Can you work these out from the model? Positions are in its coordinate system, mm. A direction names the side the tool comes from. Give positions to 0.01 mm unless a question says otherwise; leave off trailing zeros. Loops run counter-clockwise (first coordinate to the right, second up) from the corner with the lowest first, then second, coordinate; pieces in that order, holes last. Notation, with made-up numbers: (62.25, 26) -> (84.25, 26) arc R15 ccw to (84.25, 43) -> close; hole circle Ø2 at (11.25, 39). An arc over 180 degrees is marked (long way). One line per question, with ' | ' between items.
from build123d import *

# Parameters (mm, degrees)
SKETCH1_W             = 30
SKETCH1_H             = 30
SKETCH1_W_2           = 20
SKETCH1_H_2           = 20
BOSS_EXTRUDE1_DEPTH   = 20
BOSS_EXTRUDE2_START   = 20
SKETCH1_2_W           = 30
SKETCH1_2_H           = 30
SKETCH1_2_W_2         = 20
SKETCH1_2_H_2         = 20
BOSS_EXTRUDE2_DEPTH   = 10
SKETCH3_R             = 2.5
CUT_EXTRUDE1_DEPTH    = 46
SKETCH3_3_R           = 4
SKETCH3_3_R_2         = 2.5
CUT_EXTRUDE2_DEPTH    = 3
CUT_EXTRUDE3_START    = -27
SKETCH3_4_R           = 4
SKETCH3_4_R_2         = 2.5
CUT_EXTRUDE3_DEPTH    = 3
BOSS_EXTRUDE4_DEPTH   = 5
FILLET2_R             = 15
SKETCH7_R             = 2.5
CUT_EXTRUDE5_DEPTH    = 105.74180253
CRVPATTERN1_START     = -5
CRVPATTERN1_OUTLINE_R = 2.5
CRVPATTERN1_DEPTH     = 10


# Read off the part's stored shape, not the designer's step: CrvPattern1
with BuildPart() as part:
    # Sketch1 → Boss-Extrude1 (new body)
    with BuildSketch(Plane(origin=(0, 0, 0), x_dir=(1, 0, 0), z_dir=(0, 1, 0))):
        Rectangle(SKETCH1_W, SKETCH1_H)
        Rectangle(SKETCH1_W_2, SKETCH1_H_2, mode=Mode.SUBTRACT)
    extrude(amount=BOSS_EXTRUDE1_DEPTH)

    # Sketch1<2> → Boss-Extrude2 (add)
    # profile 1 of 2: a face of its own
    with BuildSketch(Plane(origin=(0, 0, 0), x_dir=(1, 0, 0), z_dir=(0, 1, 0)).offset(BOSS_EXTRUDE2_START)):
        Rectangle(SKETCH1_2_W, SKETCH1_2_H)
        Rectangle(SKETCH1_2_W_2, SKETCH1_2_H_2, mode=Mode.SUBTRACT)
    # profile 2 of 2: a face of its own
    with BuildSketch(Plane(origin=(0, 0, 0), x_dir=(1, 0, 0), z_dir=(0, 1, 0)).offset(BOSS_EXTRUDE2_START)):
        Rectangle(SKETCH1_2_W_2, SKETCH1_2_H_2)
    extrude(amount=BOSS_EXTRUDE2_DEPTH)

    # Sketch3 → Cut-Extrude1 (cut, through all)
    with BuildSketch(Plane(origin=(15, 0, 0), x_dir=(0, 0, -1), z_dir=(1, 0, 0))):
        with Locations((0, 15)):
            Circle(SKETCH3_R)
    extrude(amount=-CUT_EXTRUDE1_DEPTH, mode=Mode.SUBTRACT)

    # Sketch3<3> → Cut-Extrude2 (cut)
    # profile 1 of 2: a face of its own
    with BuildSketch(Plane(origin=(15, 0, 0), x_dir=(0, 0, -1), z_dir=(1, 0, 0))):
        Polygon((-5, 17.886751346), (-5, 12.113248654), (0, 9.226497308), (5, 12.113248654), (5, 17.886751346), (0, 20.773502692), align=None)
        with Locations((0, 15)):
            Circle(SKETCH3_3_R, mode=Mode.SUBTRACT)
    # profile 2 of 2: a face of its own
    with BuildSketch(Plane(origin=(15, 0, 0), x_dir=(0, 0, -1), z_dir=(1, 0, 0))):
        with Locations((0, 15)):
            Circle(SKETCH3_3_R)
        with Locations((0, 15)):
            Circle(SKETCH3_3_R_2, mode=Mode.SUBTRACT)
    extrude(amount=-CUT_EXTRUDE2_DEPTH, mode=Mode.SUBTRACT)

    # Sketch3<4> → Cut-Extrude3 (cut)
    with BuildSketch(Plane(origin=(15, 0, 0), x_dir=(0, 0, -1), z_dir=(1, 0, 0)).offset(CUT_EXTRUDE3_START)):
        with Locations((0, 15)):
            Circle(SKETCH3_4_R)
        with Locations((0, 15)):
            Circle(SKETCH3_4_R_2, mode=Mode.SUBTRACT)
    extrude(amount=-CUT_EXTRUDE3_DEPTH, mode=Mode.SUBTRACT)

    # Sketch6 → Boss-Extrude4 (add, symmetric)
    with BuildSketch(Plane(origin=(0, 0, 0), x_dir=(0, 0, -1), z_dir=(1, 0, 0))):
        Polygon((-15, 30), (-15, 100), (25.559724605, 100), (15, 0), (15, 30), align=None)
    extrude(amount=BOSS_EXTRUDE4_DEPTH, both=True)

    # Fillet2
    fillet2_edges = [part.edges().sort_by_distance(p)[0] for p in [
        (0, 100, -25.559724605),
        (0, 100, 15),
    ]]
    fillet(fillet2_edges, radius=FILLET2_R)

    # Sketch7 → Cut-Extrude5 (cut, through all)
    with BuildSketch(Plane(origin=(5, 0, 0), x_dir=(0, 0, -1), z_dir=(1, 0, 0))):
        with Locations((0, 40)):
            Circle(SKETCH7_R)
    extrude(amount=-CUT_EXTRUDE5_DEPTH, mode=Mode.SUBTRACT)

    # CrvPattern1 outline → CrvPattern1 (cut)
    with BuildSketch(Plane.YZ.offset(CRVPATTERN1_START)):
        with Locations((47.499218774, -0.093745117)):
            Circle(CRVPATTERN1_OUTLINE_R)
        with Locations((92.232441278, -4.582038329)):
            Circle(CRVPATTERN1_OUTLINE_R)
        with Locations((84.831439742, -3.368676619)):
            Circle(CRVPATTERN1_OUTLINE_R)
        with Locations((77.402420016, -2.340699831)):
            Circle(CRVPATTERN1_OUTLINE_R)
        with Locations((69.950024994, -1.498750417)):
            Circle(CRVPATTERN1_OUTLINE_R)
        with Locations((62.478912182, -0.843354566)):
            Circle(CRVPATTERN1_OUTLINE_R)
        with Locations((54.993750781, -0.374921882)):
            Circle(CRVPATTERN1_OUTLINE_R)
    extrude(amount=CRVPATTERN1_DEPTH, mode=Mode.SUBTRACT)


solid = part.part
Q1. If I drill on probe 1 along X at (y, z) = (11, -8); probe 2 along Y at (x, z) = (11.05, 0), over which ranges is the centre line in solid material (lowest first)? Write a range as from..to.
Entries:
probe 1: -15..-10, 10..15 | probe 2: 0..12.5, 17.5..30
Q2. If we section it at C-C (y = 7): Write out the boundary of the cut face in (x, z).
Entries:
outline: (-15, -15) -> (-5, -15) -> (-5, -15.74) -> (5, -15.74) -> (5, -15) -> (15, -15) -> (15, 15) -> (-15, 15) -> close; hole (-10, -10) -> (10, -10) -> (10, 10) -> (-10, 10) -> close
Q3. If we section it at D-D (x = 6): Write out the boundary of the cut face in (y, z).
Entries:
outline: (0, -15) -> (30, -15) -> (30, 15) -> (0, 15) -> (0, 10) -> (20, 10) -> (20, -10) -> (0, -10) -> close
Q4. If we section it at B-B (y = 40): Write out the boundary of the cut face in (x, z), plus the area to 3 significant figures.
Entries:
outline: (-5, -19.22) -> (5, -19.22) -> (5, -2.5) -> (-5, -2.5) -> close; (-5, 2.5) -> (5, 2.5) -> (5, 15) -> (-5, 15) -> close | area: 292 mm²
Q5. On a 3-axis mill with a long thin cutter (end or side, diameter ignored), from which of +Z, -Z, +X, -X, +Y, -Y can I reach the whole of each face in a straight line? I mean faces 5 (the face through (-10, 10, 0)), 6 (the face through (-0.07, 82.334, -3.259)), 7 (the face through (-13.479, 18.966, 0.521)), 8 (the face through (14, 15, 5)). Say none if no direction works.
Entries:
face 5: -Y | face 6: +X, -X | face 7: -X | face 8: +X
Q6. If we section it at A-A (x = -11): Write out the boundary of the cut face in (y, z), plus the area to 3 significant figures.
Entries:
outline: (0, -15) -> (30, -15) -> (30, 15) -> (0, 15) -> close; hole circle Ø5 at (15, 0) | area: 880 mm²
Q7. If we mould it in two halves opening along Y, with no side actions, what happens to faces 1 (the face through (10, 30, 0)), 2 (the face through (12, 12.5, 1.2)), 3 (the face through (0, 20, 0)), 4 (the face through (13.521, 10.65, -2.465))? For each: pulls with the +Y half, pulls with the -Y half, needs draft (parallel to the pull), parting line crosses it, or undercut.
Entries:
face 1: pulls with the +Y half | face 2: undercut | face 3: pulls with the -Y half | face 4: undercut
Q8. For pin 1 Ø5 at (x, y) = (-2.5, 13) entering from -Z; pin 2 Ø8 at (y, z) = (47.5, -0.09) entering from -X; pin 3 Ø12 at (y, z) = (60, -12) entering from +X; pin 4 Ø4.5 at (y, z) = (77.4, -2.34) entering from +X, each with a flat end and sliding along its axis, tell me the tip position at first contact or that it passes through.
Entries:
pin 1: z = -16.64 | pin 2: x = -5 | pin 3: x = 5 | pin 4: through
